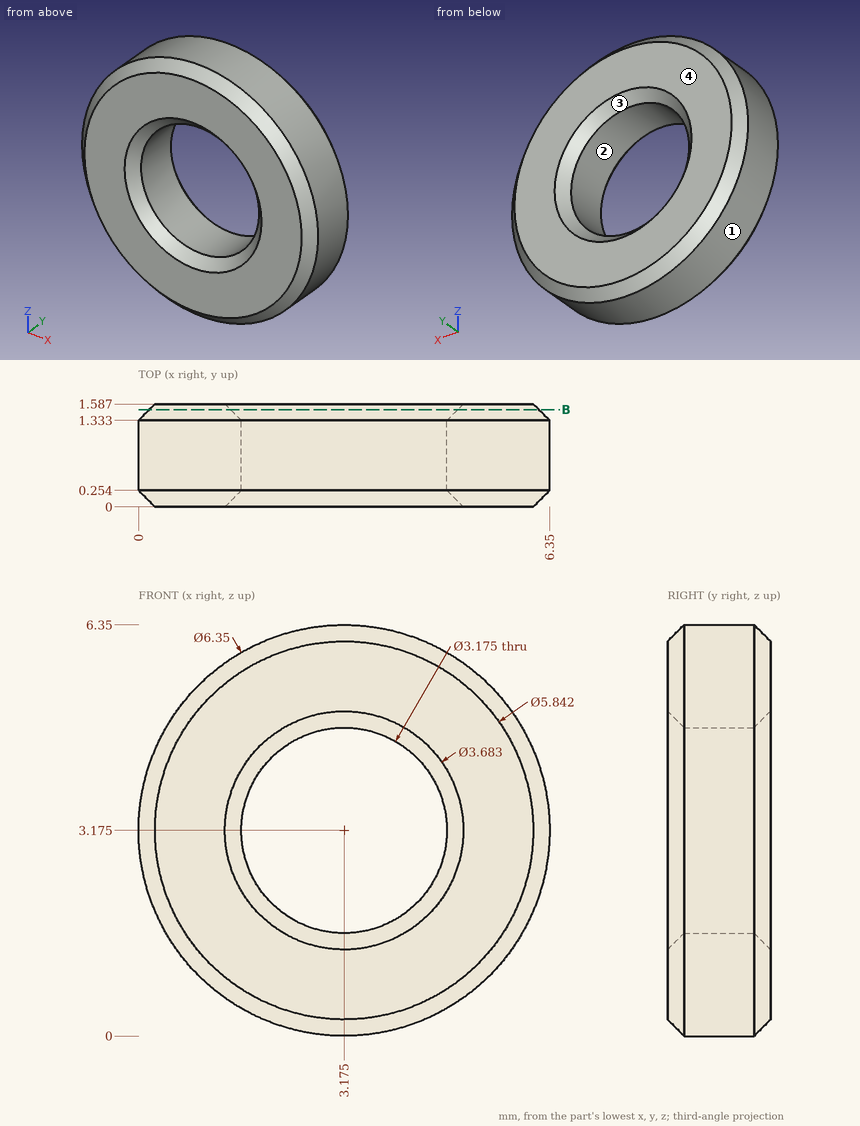
Drawing for the job (mm, zero at the part's lowest x, y, z). Round coordinates to 2 decimals unless told otherwise and drop trailing zeros. Write each loop counter-clockwise with the first axis right and the second up, starting at its lowest first coordinate (ties: lowest second). Pieces come first, ordered by that corner, then holes. Notation, with made-up numbers: (70, 45) - (115, 45) arc R21 ccw to (115, 63) - close; hole circle Ø7 at (55, 65). An arc over 180 degrees is marked (long way). Return JSON: item names as keys, results as strings. Group by question number.
Item 1: Band-saw the part on B-B on y = 1.5. List the corners of the cut face in (x, z) (1 decimal).
Item 2: Flat gauge pin, fed straight in: pin 1 Ø1.9 at (x, z) = (3.175, 3.175) entering from +Y. Where does the tip first touch, or does it go through?
Item 3: Probe probe 1 along X at (y, z) = (0.45, 1.75) (1 decimal); probe 2 along X at (y, z) = (0.6, 3.5). List the from-to ranges inside material, lowest first.
Item 4: Mould opens along X. For the marked faces 1, 2, 3 and 4 say: +X half, -X half, draft (parallel to the pull), parting line (faces both ways), or undercut.
Resolved:
{
 "1": {"outline": "circle Ø6 at (3.2, 3.2); hole circle Ø3.5 at (3.2, 3.2)"},
 "2": {"pin 1": "passes through"},
 "3": {"probe 1": "x = 0.3 to 2.5, 3.9 to 6", "probe 2": "x = 0.02 to 1.62, 4.73 to 6.33"},
 "4": {"face 1": "parting line", "face 2": "undercut", "face 3": "undercut", "face 4": "draft"}
}
